```python
from build123d import *

# Parameters (mm, degrees)
F1_DEPTH = 30.97
F2_W     = 2.25
F2_H     = 41.1360506777
F2_H_2   = 42.1689638739
F3_DEPTH = 4.15
F4_SIZE  = 1
F5_SIZE  = 1
F7_DEPTH = 85.13


with BuildPart() as f1:
    # F0 (on Right) → F1 (new body)
    with BuildSketch(Plane.YZ):
        Polygon((97.6600019388, 28.3032343221), (97.6600019388, 34.6382343221), (12.5300019388, 37.9532343221), (12.5300019388, 28.3032343221), align=None)
    extrude(amount=-F1_DEPTH)

    # F2 (on face) → F3 (join)
    with BuildSketch(Plane(origin=(0, 1.4946493439, 38.3829558521), x_dir=(1, 0, 0), z_dir=(0, 0.0389109537, 0.9992426821))):
        with Locations((-1.125, 54.6446547341)):
            Rectangle(F2_W, F2_H)
        with Locations((-29.845, 54.128198136)):
            Rectangle(F2_W, F2_H_2)
    extrude(amount=F3_DEPTH)

    # F4
    f4_edges = [f1.edges().sort_by_distance(p)[0] for p in [
        (-28.72, 55.743336, 40.423633),
        (-2.25, 56.259401, 40.403537),
    ]]
    chamfer(f4_edges, length=F4_SIZE)

    # F5
    f5_edges = [f1.edges().sort_by_distance(p)[0] for p in [
        (-2.25, 76.711654, 37.030166),
        (-2.25, 35.606757, 38.630809),
        (-28.72, 34.574626, 38.671001),
        (-28.72, 76.711654, 37.030166),
    ]]
    chamfer(f5_edges, length=F5_SIZE)

    # F6 (on face) → F7 (join, through all)
    with BuildSketch(Plane.XZ.offset(-12.5300019388)):
        with BuildLine():
            Line((0, 28.3032343221), (-30.97, 28.3032343221))
            Line((-30.97, 28.3032343221), (-30.97, 23.3032343221))
            ThreePointArc((-30.97, 23.3032343221), (-15.485, 28.1745693779), (0, 23.3032343221))
            Line((0, 23.3032343221), (0, 28.3032343221))
        make_face()
    extrude(amount=-F7_DEPTH)


solid = f1.part
```
Build history of the part. All positions in model axes, mm. A direction names the side the tool comes from. Coordinates: 2 decimals unless noted, no trailing zeros. Write each loop counter-clockwise with the first axis right and the second up, starting at its lowest first coordinate (ties: lowest second). Pieces come first, ordered by that corner, then holes.
1. Drill centre lines: probe 1 along X at (y, z) = (51.5, 36.75); probe 2 along Z at (x, y) = (-18.5, 39.5); probe 3 along Z at (x, y) = (-9.5, 62). Where is each one in solid material? Low to high.
Answer block:
probe 1: x = -30.97 to -28.72, -2.25 to 0
probe 2: z = 28.01 to 36.9
probe 3: z = 27.5 to 36.03
2. Pull direction X, two halves, no side cores. Call faces 3 (the flat face through (-16, 97.66, 30)), 4 (the cylindrical face through (-15.716, 54.499, 28.174)), 5 (the flat face through (0, 54, 30)), 6 (the flat face through (-2.25, 56, 38)): released by +X, released by -X, zero draft, split by the parting line, or undercut.
Answer block:
face 3: zero draft
face 4: undercut
face 5: released by +X
face 6: undercut
3. Band-saw the part on C-C, the plane x = -15.5. Give the cut face in (y, z).
Answer block:
outline: (12.53, 28.17) - (97.66, 28.17) - (97.66, 34.64) - (12.53, 37.95) - close
4. Band-saw the part on B-B, the plane y = 48. Give the cut face in (x, z) (3 decimals), and give its area (3 significant figures).
Answer block:
outline: (-30.97, 23.303) arc R27.048 cw to (0, 23.303) - (0, 40.725) - (-1.25, 40.725) - (-2.25, 39.724) - (-2.25, 36.572) - (-28.72, 36.572) - (-28.72, 39.724) - (-29.72, 40.725) - (-30.97, 40.725) - close
area: 326 mm2
5. Drop flat-ended pins along their axis: pin 1 (5 mm diameter, centred on x = -4.5, y = 27, fed in from +Z); pin 2 (2 mm diameter, centred on x = -16.5, y = 78.5, fed in from +Z); pin 3 (8 mm diameter, centred on x = -24.5, y = 74, fed in from -Z). Give the stop position or say it passes through.
Answer block:
pin 1: stops at z = 37.49
pin 2: stops at z = 35.42
pin 3: stops at z = 24.84
6. Band-saw the part on A-A, the plane z = 27. Give the cut face in (x, y), and give its area (3 significant figures).
Answer block:
outline: (-30.97, 12.53) - (-23.37, 12.53) - (-23.37, 97.66) - (-30.97, 97.66) - close; (-7.6, 12.53) - (0, 12.53) - (0, 97.66) - (-7.6, 97.66) - close
area: 1,290 mm2
7. 3-axis set-ups, long thin cutter, end or side, ignore diameter. For faces 1 (the flat face through (-28.72, 55, 38)), 2 (the flat face through (-16, 12.53, 32)): which of +Z, -Z, +X, -X, +Y, -Y reach the whole face in a straight line?
Answer block:
face 1: +Z, +Y
face 2: +Z, -Z, +X, -X, -Y
8. Band-saw the part on D-D, the plane y = 62.5. Give the cut face in (x, z) (3 decimals), and give its area (3 significant figures).
Answer block:
outline: (-30.97, 23.303) arc R27.048 cw to (0, 23.303) - (0, 40.161) - (-1.25, 40.161) - (-2.25, 39.16) - (-2.25, 36.007) - (-28.72, 36.007) - (-28.72, 39.16) - (-29.72, 40.161) - (-30.97, 40.161) - close
area: 309 mm2
